Build history of the part. All positions in model axes, mm. Give positions to 0.01 mm unless a question says otherwise; leave off trailing zeros. Order: outer loops, then holes, each group sorted by start corner. A loop starts at its lowest first (then second) coordinate and runs counter-clockwise, first axis right, second up. Notation, with made-up numbers: (-2.75, 62) - (41.25, 62) arc R32 cw to (41.25, 101) - close; hole circle Ø8 at (36.25, 5.25). An arc over 180 degrees is marked (long way). Use a Markdown table: item, result. Add a question column.
(1) Slice it at C-C (y = 1.9). Write the cut outline in (x, z).
(2) Slice it at B-B (z = 0.5). Write the cut outline in (x, y).
(3) Slice it at D-D (x = -1.25). Write the cut outline in (y, z).
(4) Flat gauge pins, fed straight in: pin 1 (1.5 mm diameter, centred on y = 1.5, z = -3, fed in from -X); pin 2 (1 mm diameter, centred on x = -1.5, y = 0.5, fed in from -Z). Where does each tip first touch, or does it go through?
(5) Wall check: line 1 (X direction, y = 1.3, z = 0); line 2 (X direction, y = 0.9, z = 1.25); line 3 (Z direction, x = -1, y = 0.3). Give the ranges that are in metal, low to high.
(6) Slice it at A-A (x = 0.5). Write the cut outline in (y, z).
Autodesk Inventor part; units mm, degrees
ref_plane "YZ Plane" through (0, 0, 0) normal (1, 0, 0) x (0, 1, 0)
ref_plane "XZ Plane" through (0, 0, 0) normal (0, 1, 0) x (-1, 0, 0)
ref_plane "XY Plane" through (0, 0, 0) normal (0, 0, 1) x (1, 0, 0)
sketch "Sketch1" plane through (0, 0, 0) normal (0, 1, 0) x (-1, 0, 0)
  circle A0 centre (0, 0) radius 2.05
  arc A1 (0, 4.35) -> (-4.35, 0) centre (0, 0) ccw construction
  line L0 (0, 4.35) -> (4.35, 4.35)
  line L1 (4.35, 0) -> (4.35, 4.35)
  line L2 (0, 4.35) -> (-4.35, 4.35)
  line L3 (-4.35, 0) -> (-4.35, 4.35)
  arc A2 (4.35, 0) -> (0, 4.35) centre (0, 0) ccw construction
  arc A3 (-4.35, 0) -> (4.35, 0) centre (0, 0) ccw
  dimension "d0" = 4.1
  dimension "d1" = 2.3
extrude "Extrusion1" add sketch "Sketch1" along normal blind 3
fillet "Fillet1" radius 3 1 edges at (-2.175, 0, 4.35)
properties part number "top_housing_screw_spacers"
Solution:
| question | item | result |
|---|---|---|
| 1 | outline | (-4.35, 0) arc R4.35 ccw to (4.35, 0) - (4.35, 4.14) - (-4.35, 4.14) - close; hole circle Ø4.1 at (0, 0) |
| 2 | outline | (-4.35, 0) - (-1.99, 0) - (-1.99, 3) - (-4.35, 3) - close; (1.99, 0) - (4.35, 0) - (4.35, 3) - (1.99, 3) - close |
| 3 | outline | (0, -4.17) - (3, -4.17) - (3, -1.62) - (0, -1.62) - close; (0.01, 1.62) - (3, 1.62) - (3, 4.35) arc R3 ccw to start |
| 4 | pin 1 | x = -3.72 |
| 4 | pin 2 | z = -4.23 |
| 5 | line 1 | -4.35 to -2.05, 2.05 to 4.35 |
| 5 | line 2 | -4.35 to -1.62, 1.62 to 4.35 |
| 5 | line 3 | -4.23 to -1.79, 1.79 to 2.66 |
| 6 | outline | (0, -4.32) - (3, -4.32) - (3, -1.99) - (0, -1.99) - close; (0.07, 1.99) - (3, 1.99) - (3, 4.35) arc R3 ccw to start |
